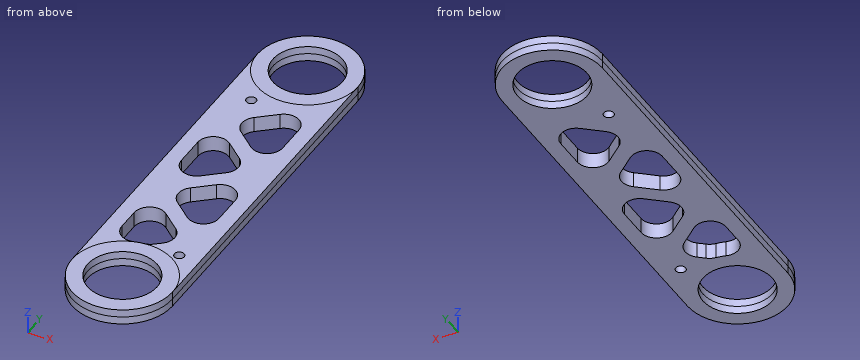
from build123d import *

# Parameters (mm, degrees)
SKETCH2_R               = 20.6375
SKETCH2_R_2             = 14.2875
BOSS_EXTRUDE1_DEPTH     = 3.175
CUT_EXTRUDE1_DEPTH      = 162.691375582
CUT_EXTRUDE1_DEPTH_BACK = 162.691375582
SKETCH3_R               = 2.0193
FILLET2_R               = 6.35


with BuildPart() as part:
    # Sketch2 → Boss-Extrude1 (new, symmetric)
    # profile 1 of 3: a face of its own
    with BuildSketch(Plane.XY):
        with BuildLine():
            Line((20.6375, 0), (20.6375, 139.7))
            ThreePointArc((20.6375, 139.7), (0, 119.0625), (-20.6375, 139.7))
            Line((-20.6375, 139.7), (-20.6375, 0))
            ThreePointArc((-20.6375, 0), (0, 20.6375), (20.6375, 0))
        make_face()
    # profile 2 of 3: a face of its own
    with BuildSketch(Plane.XY):
        with Locations((0, 139.7)):
            Circle(SKETCH2_R)
        with Locations((0, 139.7)):
            Circle(SKETCH2_R_2, mode=Mode.SUBTRACT)
    # profile 3 of 3: a face of its own
    with BuildSketch(Plane.XY):
        Circle(SKETCH2_R)
        Circle(SKETCH2_R_2, mode=Mode.SUBTRACT)
    extrude(amount=BOSS_EXTRUDE1_DEPTH, both=True)

    # Sketch3 → Cut-Extrude1 (cut, two sides: drawn at the far end of the back side and taken through both)
    with BuildSketch(Plane.XY.offset(-CUT_EXTRUDE1_DEPTH_BACK)):
        Polygon((14.2875, 80.998054184), (14.2875, 120.663261819), (-9.34807685, 100.830658002), align=None)
        Polygon((9.34807685, 76.853386041), (-14.2875, 96.685989858), (-14.2875, 57.020782224), align=None)
        Polygon((14.2875, 33.043510263), (14.2875, 72.708717897), (-9.34807685, 52.87611408), align=None)
        with BuildLine():
            Line((9.34807685, 28.898842119), (-14.2875, 48.731445936))
            Line((-14.2875, 48.731445936), (-14.2875, 14.892070037))
            ThreePointArc((-14.2875, 14.892070037), (-7.933318425, 19.051741785), (-0.504765013, 20.631326146))
            Line((-0.504765013, 20.631326146), (9.34807685, 28.898842119))
        make_face()
        with Locations((-9.34807685, 114.324408002)):
            Circle(SKETCH3_R)
        with Locations((12.2682, 20.423771151)):
            Circle(SKETCH3_R)
    extrude(amount=CUT_EXTRUDE1_DEPTH + CUT_EXTRUDE1_DEPTH_BACK, mode=Mode.SUBTRACT)

    # Fillet2
    fillet2_edges = [part.edges().sort_by_distance(p)[0] for p in [
        (-0.504765013, 20.631326146, 0),
        (-14.2875, 14.892070037, 0),
        (-14.2875, 48.731445936, 0),
        (9.34807685, 28.898842119, 0),
        (9.34807685, 76.853386041, 0),
        (-14.2875, 57.020782224, 0),
        (-14.2875, 96.685989858, 0),
        (-9.34807685, 52.87611408, 0),
        (14.2875, 72.708717897, 0),
        (14.2875, 33.043510263, 0),
        (-9.34807685, 100.830658002, 0),
        (14.2875, 120.663261819, 0),
        (14.2875, 80.998054184, 0),
    ]]
    fillet(fillet2_edges, radius=FILLET2_R)


solid = part.part
Part model, mm, in its own coordinate system. Give positions to 0.01 mm unless a question says otherwise; leave off trailing zeros. Order: outer loops, then holes, each group sorted by start corner. A loop starts at its lowest first (then second) coordinate and runs counter-clockwise, first axis right, second up. Notation, with made-up numbers: (-15.5, -1.5) - (-3.5, -1.5) arc R21 cw to (-3.5, 25.5) - close; hole circle Ø10 at (-21.75, 78.25). An arc over 180 degrees is marked (long way). One line per question, with ' | ' between items.
1. Band-saw the part on A-A on x = 8. List the corners of the cut face in (y, z) (3 decimals), then the cut area to 3 significant figures.
Filled in:
outline: (-19.024, -3.175) - (-11.838, -3.175) - (-11.838, 3.175) - (-19.024, 3.175) - close; (11.838, -3.175) - (40.311, -3.175) - (40.311, 3.175) - (11.838, 3.175) - close; (65.441, -3.175) - (88.266, -3.175) - (88.266, 3.175) - (65.441, 3.175) - close; (113.395, -3.175) - (127.862, -3.175) - (127.862, 3.175) - (113.395, 3.175) - close; (151.538, -3.175) - (158.724, -3.175) - (158.724, 3.175) - (151.538, 3.175) - close | area: 509 mm²
2. Band-saw the part on D-D on y = 110. List the corners of the cut face in (x, z) (1 decimal), then the cut area to 3 significant figures.
Filled in:
outline: (-20.6, -3.2) - (1.6, -3.2) - (1.6, 3.2) - (-20.6, 3.2) - close; (13.6, -3.2) - (20.6, -3.2) - (20.6, 3.2) - (13.6, 3.2) - close | area: 186 mm²
3. Band-saw the part on B-B on y = -3. List the corners of the cut face in (x, z) (3 decimals).
Filled in:
outline: (-20.418, -3.175) - (-13.969, -3.175) - (-13.969, 3.175) - (-20.418, 3.175) - close; (13.969, -3.175) - (20.418, -3.175) - (20.418, 3.175) - (13.969, 3.175) - close
4. Drill centre lines: probe 1 along Y at (x, z) = (-7.5, 1.5); probe 2 along Y at (x, z) = (-7, -1.5); probe 3 along X at (y, z) = (80, 1.25). Where is each one in solid material? Low to high.
Filled in:
probe 1: -19.23 to -12.16, 12.16 to 19.46, 41.45 to 64.3, 89.4 to 113.51, 115.14 to 127.54, 151.86 to 158.93 | probe 2: -19.41 to -12.46, 12.46 to 19.51, 41.39 to 64.36, 89.35 to 127.24, 152.16 to 159.11 | probe 3: -20.64 to -14.29, 4.98 to 20.64
5. Drop flat-ended pins along their axis: P1, Ø1, axis at x = 6, z = -2, coming from the +Y side; P2, Ø8, axis at x = 6.5, y = 133, coming from the +Z side; P3, Ø2, axis at x = 0, z = -1.5, coming from the -Y side; P4, Ø1, axis at x = 9, z = 0, coming from the +Y side. Give the stop position or say it passes through.
Filled in:
P1: y = 159.59 | P2: through | P3: y = -20.64 | P4: y = 158.51
6. Band-saw the part on C-C on x = -9. List the corners of the cut face in (y, z) (3 decimals).
Filled in:
outline: (-18.572, -3.175) - (-11.097, -3.175) - (-11.097, 3.175) - (-18.572, 3.175) - close; (11.097, -3.175) - (19.533, -3.175) - (19.533, 3.175) - (11.097, 3.175) - close; (41.374, -3.175) - (64.378, -3.175) - (64.378, 3.175) - (41.374, 3.175) - close; (89.329, -3.175) - (112.335, -3.175) - (112.335, 3.175) - (89.329, 3.175) - close; (116.313, -3.175) - (128.603, -3.175) - (128.603, 3.175) - (116.313, 3.175) - close; (150.797, -3.175) - (158.272, -3.175) - (158.272, 3.175) - (150.797, 3.175) - close
